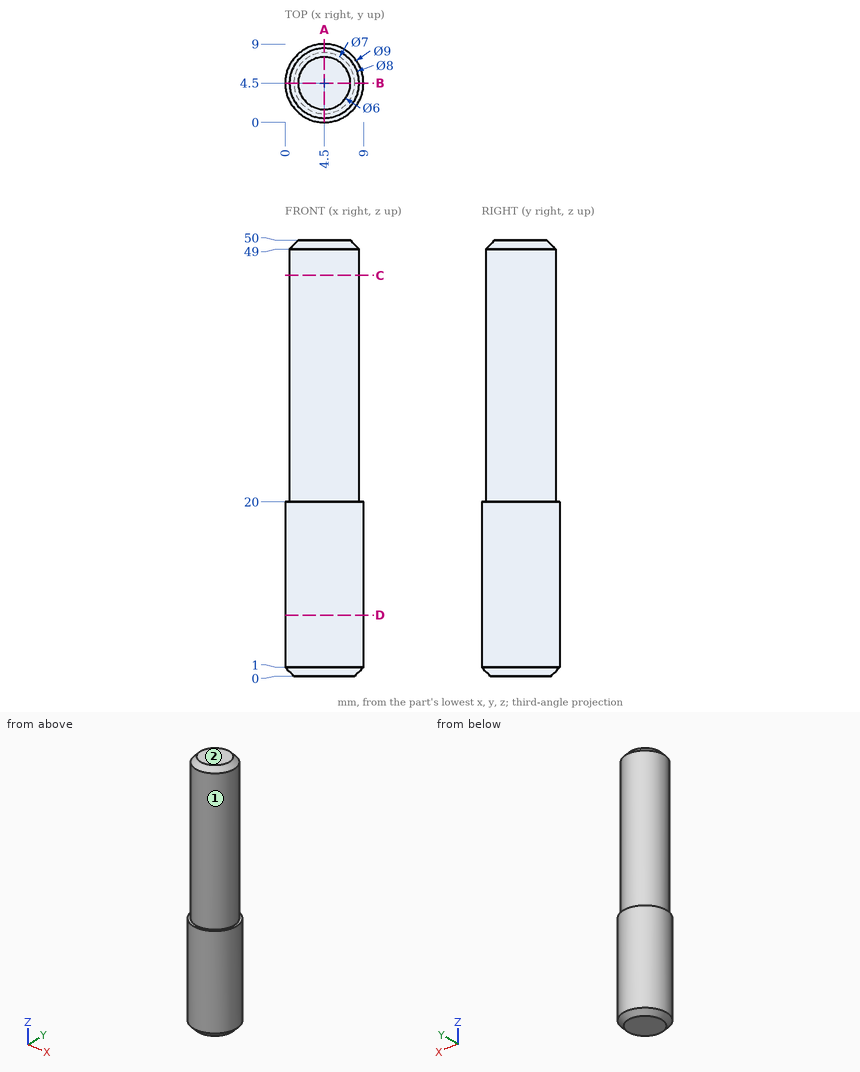
Answer from the drawing. Dimensions are ordinates in mm from the lowest x, y and z of the part. A direction names the side the tool comes from. Coordinates: 2 decimals unless noted, no trailing zeros. Order: outer loops, then holes, each group sorted by start corner. A loop starts at its lowest first (then second) coordinate and runs counter-clockwise, first axis right, second up. Notation, with made-up numbers: (25.5, -14.5) - (64.5, -14.5) arc R16 cw to (64.5, 14.5) - close; hole circle Ø6 at (56.25, 85.25). An arc over 180 degrees is marked (long way). Use one line per item in the form item = value.
(1) Given pin 1 Ø5 at (y, z) = (2.5, 43) entering from +X; pin 2 Ø2 at (y, z) = (8, 31) entering from +X, each flat-ended and moving along its own axis, determine where each tip first touches the part or whether it passes through.
Computed values:
pin_1 = 8.5
pin_2 = 7.62
(2) Section D-D, the plane z = 7 is taken. Give the vertices of the cut face in (x, y).
Computed values:
outline = circle Ø9 at (4.5, 4.5)
(3) Straight lines are drawn through the part: L1, parallel to Y at x = 6.75, z = 25; L2, parallel to X at y = 2.5, z = 40; L3, parallel to Y at x = 3.5, z = 43. For each, find the intervals that lie inside material, in ascending order.
Computed values:
L1 = 1.19 to 7.81
L2 = 1.04 to 7.96
L3 = 0.63 to 8.37
(4) Section A-A, the plane x = 4.5 is taken. Give the vertices of the cut face in (y, z).
Computed values:
outline = (0, 1) - (1, 0) - (8, 0) - (9, 1) - (9, 20) - (8.5, 20) - (8.5, 49) - (7.5, 50) - (1.5, 50) - (0.5, 49) - (0.5, 20) - (0, 20) - close
(5) Section C-C, the plane z = 46 is taken. Give the vertices of the cut face in (x, y).
Computed values:
outline = circle Ø8 at (4.5, 4.5)
(6) Which of the six approach directions +Z, -Z, +X, -X, +Y, -Y give full straight-line access (tool end or side, diameter ignored) to the marked faces 1 and 2?
Computed values:
face_1 = +Z
face_2 = +Z, +X, -X, +Y, -Y
